from build123d import *

# Parameters (mm, degrees)
F0_W          = 30
F0_H          = 30
F4_DEPTH      = 3
F3_W          = 30
F3_H          = 30
F5_DEPTH      = 8
F6_DEPTH      = 25
F8_DEPTH      = 6.0000000522
F10_DEPTH     = 30
F7_W          = 10
F7_H          = 11.7721162952
F7_H_2        = 1.030384494
F11_DEPTH     = 35.21044533
F12_T4_DEPTH  = 18.4976166065
F12_T10_DEPTH = 18.4976166065
F12_T15_DEPTH = 17.5385665297
F12_T20_DEPTH = 17.5385665297
F12_T26_DEPTH = 17.5385665297
F12_T31_DEPTH = 17.5385665297
F12_T37_DEPTH = 18.4976166065
F12_T43_DEPTH = 18.4976166065
F12_T45_DEPTH = 13.9174578279
F12_T47_DEPTH = 24
F12_T49_DEPTH = 44.997612514
F12_T54_DEPTH = 3
F12_T60_DEPTH = 3
F3_W_2        = 10
F3_H_2        = 13
F13_DEPTH     = 5.1313021672
F14_DEPTH     = 10.5


# Not quite as in the source:
# - a fillet or chamfer that OpenCascade refuses, or shapes differently, is made with other operations: its cross-section is extruded or revolved along the edge and cut away or added


with BuildPart() as f4:
    # F0 (on Top) → F4 (new body)
    with BuildSketch(Plane.XY):
        with Locations((0, 15)):
            Rectangle(F0_W, F0_H)
    extrude(amount=F4_DEPTH)

    # F3 (on 3pt) → F5 (join)
    with BuildSketch(Plane(origin=(0, 0, 0), x_dir=(-1, 0, 0), z_dir=(0, 0.984807753, 0.1736481777))):
        with Locations((0, 15)):
            Rectangle(F3_W, F3_H)
        Polygon((-14, 2), (-14, 15), (-14, 25), (14, 25), (14, 2), (-4, 2), align=None, mode=Mode.SUBTRACT)
        Polygon((-14, 25), (-14, 15), (-4, 15), (-4, 2), (14, 2), (14, 25), align=None)
    extrude(amount=F5_DEPTH)

    # F0 (on Top) → F6 (cut)
    with BuildSketch(Plane.XY):
        with Locations((0, 15)):
            Rectangle(F0_W, F0_H)
    extrude(amount=-F6_DEPTH, mode=Mode.SUBTRACT)

    # F3 (on 3pt) → F8 (cut)
    with BuildSketch(Plane(origin=(0, 0, 0), x_dir=(-1, 0, 0), z_dir=(0, 0.984807753, 0.1736481777))):
        Polygon((-14, 25), (-14, 15), (-4, 15), (-4, 2), (14, 2), (14, 25), align=None)
    extrude(amount=F8_DEPTH, mode=Mode.SUBTRACT)

    # F9 (on face) → F10 (join, through all)
    with BuildSketch(Plane.YZ.offset(15)):
        Polygon((30, 3), (2.6690166941, 30.9334180117), (7.594431953, 3), align=None)
        with BuildLine():
            ThreePointArc((11.3703802933, 5.5), (10.0848050739, 5.9679111138), (9.4007647872, 7.1527036447))
            Line((9.4007647872, 7.1527036447), (7.6573020205, 17.0403723366))
            ThreePointArc((7.6573020205, 17.0403723366), (8.7131028501, 19.1666972856), (11.0564624317, 18.7863828744))
            Line((11.0564624317, 18.7863828744), (20.7308856563, 8.8987141825))
            ThreePointArc((20.7308856563, 8.8987141825), (21.1449009434, 6.7245737833), (19.3013407511, 5.5))
            Line((19.3013407511, 5.5), (11.3703802933, 5.5))
        make_face(mode=Mode.SUBTRACT)
    extrude(amount=-F10_DEPTH)

    # F7 (on face) → F11 (cut, through all)
    with BuildSketch(Plane(origin=(0, 30, 0), x_dir=(-1, 0, 0), z_dir=(0, 1, 0))):
        with Locations((-9, 8.8860581476)):
            Rectangle(F7_W, F7_H)
        with Locations((-9, 2.484807753)):
            Rectangle(F7_W, F7_H_2)
    extrude(amount=-F11_DEPTH, mode=Mode.SUBTRACT)

    # F12: fillet of radius 3 on 9 edges, made by hand


with BuildPart() as f12_tool2:
    # F12_s3 → F12_t4 (new body)
    with BuildSketch(Plane.XZ.offset(-25.9817706947)):
        with BuildLine():
            ThreePointArc((7, 14.7721162952), (4.8786796564, 13.8934366387), (4, 11.7721162952))
            Line((4, 11.7721162952), (4, 14.7721162952))
            Line((4, 14.7721162952), (7, 14.7721162952))
        make_face()
    extrude(amount=F12_T4_DEPTH)

    split(bisect_by=Plane(origin=(0, 16.8266333185, 16.4637365227), x_dir=(1, 0, 0), z_dir=(0, -0.7147724526, -0.6993570912)), keep=Keep.TOP)

    split(bisect_by=Plane(origin=(0, 15.0397021871, 14.7153437946), x_dir=(1, 0, 0), z_dir=(0, 0.7147724526, 0.6993570912)), keep=Keep.TOP)


with BuildPart() as f4_1:
    add(f4.part)

    # F12_t1: union F12_tool2
    add(f12_tool2.part)


with BuildPart() as f12_tool8:
    # F12_s9 → F12_t10 (new body)
    with BuildSketch(Plane.XZ.offset(-25.9817706947)):
        with BuildLine():
            ThreePointArc((7, 14.7721162952), (4.8786796564, 13.8934366387), (4, 11.7721162952))
            Line((4, 11.7721162952), (4, 14.7721162952))
            Line((4, 14.7721162952), (7, 14.7721162952))
        make_face()
    extrude(amount=F12_T10_DEPTH)

    split(bisect_by=Plane(origin=(0, 10.3404814066, 1.8233058655), x_dir=(1, 0, 0), z_dir=(0, -0.984807753, -0.1736481777)), keep=Keep.TOP)


with BuildPart() as f4_2:
    add(f4_1.part)

    # F12_t7: union F12_tool8
    add(f12_tool8.part)


with BuildPart() as f12_tool13:
    # F12_s14 → F12_t15 (new body)
    with BuildSketch(Plane.XZ.offset(-15.5572567598)):
        with BuildLine():
            ThreePointArc((7, 14.7721162952), (4.8786796564, 13.8934366387), (4, 11.7721162952))
            Line((4, 11.7721162952), (4, 14.7721162952))
            Line((4, 14.7721162952), (7, 14.7721162952))
        make_face()
    extrude(amount=F12_T15_DEPTH)

    split(bisect_by=Plane(origin=(0, 15.0397021871, 14.7153437946), x_dir=(1, 0, 0), z_dir=(0, 0.7147724526, 0.6993570912)), keep=Keep.TOP)


with BuildPart() as f4_3:
    add(f4_2.part)

    # F12_t12: union F12_tool13
    add(f12_tool13.part)


with BuildPart() as f12_tool18:
    # F12_s19 → F12_t20 (new body)
    with BuildSketch(Plane.XZ.offset(-15.5572567598)):
        with BuildLine():
            ThreePointArc((7, 14.7721162952), (4.8786796564, 13.8934366387), (4, 11.7721162952))
            Line((4, 11.7721162952), (4, 14.7721162952))
            Line((4, 14.7721162952), (7, 14.7721162952))
        make_face()
    extrude(amount=F12_T20_DEPTH)

    split(bisect_by=Plane(origin=(0, 10.3404814066, 1.8233058655), x_dir=(1, 0, 0), z_dir=(0, -0.984807753, -0.1736481777)), keep=Keep.TOP)

    split(bisect_by=Plane(origin=(0, 7.8784620241, 1.3891854213), x_dir=(1, 0, 0), z_dir=(0, 0.984807753, 0.1736481777)), keep=Keep.TOP)


with BuildPart() as f4_4:
    add(f4_3.part)

    # F12_t17: union F12_tool18
    add(f12_tool18.part)


with BuildPart() as f12_tool24:
    # F12_s25 → F12_t26 (new body)
    with BuildSketch(Plane.XZ.offset(-15.5572567598)):
        with BuildLine():
            ThreePointArc((14, 11.7721162952), (13.1213203436, 13.8934366387), (11, 14.7721162952))
            Line((11, 14.7721162952), (14, 14.7721162952))
            Line((14, 14.7721162952), (14, 11.7721162952))
        make_face()
    extrude(amount=F12_T26_DEPTH)

    split(bisect_by=Plane(origin=(0, 15.0397021871, 14.7153437946), x_dir=(1, 0, 0), z_dir=(0, 0.7147724526, 0.6993570912)), keep=Keep.TOP)


with BuildPart() as f4_5:
    add(f4_4.part)

    # F12_t23: union F12_tool24
    add(f12_tool24.part)


with BuildPart() as f12_tool29:
    # F12_s30 → F12_t31 (new body)
    with BuildSketch(Plane.XZ.offset(-15.5572567598)):
        with BuildLine():
            ThreePointArc((14, 11.7721162952), (13.1213203436, 13.8934366387), (11, 14.7721162952))
            Line((11, 14.7721162952), (14, 14.7721162952))
            Line((14, 14.7721162952), (14, 11.7721162952))
        make_face()
    extrude(amount=F12_T31_DEPTH)

    split(bisect_by=Plane(origin=(0, 10.3404814066, 1.8233058655), x_dir=(1, 0, 0), z_dir=(0, -0.984807753, -0.1736481777)), keep=Keep.TOP)

    split(bisect_by=Plane(origin=(0, 7.8784620241, 1.3891854213), x_dir=(1, 0, 0), z_dir=(0, 0.984807753, 0.1736481777)), keep=Keep.TOP)


with BuildPart() as f4_6:
    add(f4_5.part)

    # F12_t28: union F12_tool29
    add(f12_tool29.part)


with BuildPart() as f12_tool35:
    # F12_s36 → F12_t37 (new body)
    with BuildSketch(Plane.XZ.offset(-25.9817706947)):
        with BuildLine():
            ThreePointArc((14, 11.7721162952), (13.1213203436, 13.8934366387), (11, 14.7721162952))
            Line((11, 14.7721162952), (14, 14.7721162952))
            Line((14, 14.7721162952), (14, 11.7721162952))
        make_face()
    extrude(amount=F12_T37_DEPTH)

    split(bisect_by=Plane(origin=(0, 16.8266333185, 16.4637365227), x_dir=(1, 0, 0), z_dir=(0, -0.7147724526, -0.6993570912)), keep=Keep.TOP)

    split(bisect_by=Plane(origin=(0, 15.0397021871, 14.7153437946), x_dir=(1, 0, 0), z_dir=(0, 0.7147724526, 0.6993570912)), keep=Keep.TOP)


with BuildPart() as f4_7:
    add(f4_6.part)

    # F12_t34: union F12_tool35
    add(f12_tool35.part)


with BuildPart() as f12_tool41:
    # F12_s42 → F12_t43 (new body)
    with BuildSketch(Plane.XZ.offset(-25.9817706947)):
        with BuildLine():
            ThreePointArc((14, 11.7721162952), (13.1213203436, 13.8934366387), (11, 14.7721162952))
            Line((11, 14.7721162952), (14, 14.7721162952))
            Line((14, 14.7721162952), (14, 11.7721162952))
        make_face()
    extrude(amount=F12_T43_DEPTH)

    split(bisect_by=Plane(origin=(0, 10.3404814066, 1.8233058655), x_dir=(1, 0, 0), z_dir=(0, -0.984807753, -0.1736481777)), keep=Keep.TOP)


with BuildPart() as f4_8:
    add(f4_7.part)

    # F12_t40: union F12_tool41
    add(f12_tool41.part)

    # F12_s46 → F12_t45 (cut)
    with BuildSketch(Plane(origin=(0, -7.3860581476, -1.3023613325), x_dir=(1, 0, 0), z_dir=(0, 0.984807753, 0.1736481777))):
        with BuildLine():
            ThreePointArc((-15, -27), (-14.1213203436, -29.1213203436), (-12, -30))
            Line((-12, -30), (-15, -30))
            Line((-15, -30), (-15, -27))
        make_face()
        with BuildLine():
            ThreePointArc((15, -27), (14.1213203436, -29.1213203436), (12, -30))
            Line((12, -30), (15, -30))
            Line((15, -30), (15, -27))
        make_face()
    extrude(amount=F12_T45_DEPTH, mode=Mode.SUBTRACT)

    # F12_s48 → F12_t47 (cut)
    with BuildSketch(Plane.YZ.offset(-12)):
        with BuildLine():
            ThreePointArc((1.1105168936, 30.6586124474), (2.5491593686, 30.5603807939), (3.7757787843, 29.8022604621))
            Line((3.7757787843, 29.8022604621), (2.6690166941, 30.9334180117))
            Line((2.6690166941, 30.9334180117), (1.1105168936, 30.6586124474))
        make_face()
    extrude(amount=F12_T47_DEPTH, mode=Mode.SUBTRACT)

    # F12_s50 → F12_t49 (cut)
    with BuildSketch(Plane(origin=(0, 18.4185448657, -18.8245299169), x_dir=(1, 0, 0), z_dir=(0, -0.6993570912, 0.7147724526))):
        with BuildLine():
            ThreePointArc((-15, 20.5412448507), (-14.1213203436, 22.6625651943), (-12, 23.5412448507))
            Line((-12, 23.5412448507), (-15, 23.5412448507))
            Line((-15, 23.5412448507), (-15, 20.5412448507))
        make_face()
        with BuildLine():
            ThreePointArc((15, 20.5412448507), (14.1213203436, 22.6625651943), (12, 23.5412448507))
            Line((12, 23.5412448507), (15, 23.5412448507))
            Line((15, 23.5412448507), (15, 20.5412448507))
        make_face()
    extrude(amount=F12_T49_DEPTH, mode=Mode.SUBTRACT)


with BuildPart() as f12_tool52:
    # F12_s53 → F12_t54 (new body)
    with BuildSketch(Plane.YZ.offset(-12)):
        Polygon((1.6314614266, 27.7041891884), (1.1105168936, 30.6586124474), (2.6690166941, 30.9334180117), (3.7757787843, 29.8022604621), align=None)
    extrude(amount=-F12_T54_DEPTH)

    # F12_s55 → F12_t56 (revolve, cut)
    with BuildSketch(Plane(origin=(-12, 1.6314614266, 27.7041891884), x_dir=(0, -0.305899314, -0.9520638685), z_dir=(0, 0.9520638685, -0.305899314))):
        with BuildLine():
            ThreePointArc((0, -3), (3, 0), (0, 3))
            Line((0, 3), (0, -3))
        make_face()
    revolve(axis=Axis((-12, 1.6314614266, 27.7041891884), (-1, 0, 0)), mode=Mode.SUBTRACT)


with BuildPart() as f4_9:
    add(f4_8.part)

    # F12_t51: cut F12_tool52
    add(f12_tool52.part, mode=Mode.SUBTRACT)


with BuildPart() as f12_tool58:
    # F12_s59 → F12_t60 (new body)
    with BuildSketch(Plane.YZ.offset(12)):
        Polygon((1.6314614266, 27.7041891884), (3.7757787843, 29.8022604621), (2.6690166941, 30.9334180117), (1.1105168936, 30.6586124474), align=None)
    extrude(amount=F12_T60_DEPTH)

    # F12_s61 → F12_t62 (revolve, cut)
    with BuildSketch(Plane(origin=(12, 1.6314614266, 27.7041891884), x_dir=(0, -0.305899314, -0.9520638685), z_dir=(0, -0.9520638685, 0.305899314))):
        with BuildLine():
            ThreePointArc((0, -3), (3, 0), (0, 3))
            Line((0, 3), (0, -3))
        make_face()
    revolve(axis=Axis((12, 1.6314614266, 27.7041891884), (1, 0, 0)), mode=Mode.SUBTRACT)


with BuildPart() as f4_10:
    add(f4_9.part)

    # F12_t57: cut F12_tool58
    add(f12_tool58.part, mode=Mode.SUBTRACT)

    # F3 (on 3pt) → F13 (cut, through all)
    with BuildSketch(Plane(origin=(0, 0, 0), x_dir=(-1, 0, 0), z_dir=(0, 0.984807753, 0.1736481777))):
        with Locations((0, 15)):
            Rectangle(F3_W, F3_H)
        Polygon((-14, 2), (-14, 15), (-14, 25), (14, 25), (14, 2), (-4, 2), align=None, mode=Mode.SUBTRACT)
        Polygon((-14, 25), (-14, 15), (-4, 15), (-4, 2), (14, 2), (14, 25), align=None)
        with Locations((-9, 8.5)):
            Rectangle(F3_W_2, F3_H_2)
    extrude(amount=-F13_DEPTH, mode=Mode.SUBTRACT)

    # F3 (on 3pt) → F14 (cut, through all)
    with BuildSketch(Plane(origin=(0, 0, 0), x_dir=(-1, 0, 0), z_dir=(0, 0.984807753, 0.1736481777))):
        with Locations((-9, 8.5)):
            Rectangle(F3_W_2, F3_H_2)
    extrude(amount=F14_DEPTH, mode=Mode.SUBTRACT)


solid = f4_10.part
Can you work these out from the model? Positions are in its coordinate system, mm. A direction names the side the tool comes from. Give positions to 0.01 mm unless a question says otherwise; leave off trailing zeros. Loops run counter-clockwise (first coordinate to the right, second up) from the corner with the lowest first, then second, coordinate; pieces in that order, holes last. Notation, with made-up numbers: M 16,-5 L 45,-5 A13 ccw 45,17 Z; hole C 49.25,-36.5 d10. An arc over 180 degrees is marked long. One line per item, written item: value.
1) Thinking about a two-plate mould opening in X: for faces 4 (the face through (-0.168, 2.53, 30.567)), 5 (the face through (9.1, 5.5, 16.2)), 6 (the face through (-15, 8, 11)), which applies, +X half, -X half, draft (parallel to the pull), parting line (faces both ways), or undercut?
Geometry check:
face 4: draft
face 5: undercut
face 6: -X half
2) Imagine slicing it at A-A on x = 9.5. Write out the boundary of the cut face in (y, z).
Geometry check:
outline: M -5.21,29.54 L -4.34,24.62 L 1.57,25.66 L 3.3,15.81 L 7.74,16.6 L 7.66,17.04 A2 cw 11.06,18.79 L 14.98,14.77 L 18.48,14.77 L 3.78,29.8 A3 ccw 1.11,30.66 Z; M -0.35,1.97 L 0,0 L 30,0 L 30,1.97 Z
3) Please list where these lines run through material, in increasing order: line 1 (X direction, y = -0.5, z = 16.5); line 2 (Z direction, x = -5.5, y = 19.5); line 3 (Z direction, x = -5, y = 15).
Geometry check:
line 1: x = -15 to -14, 14 to 15
line 2: z = 0 to 5.51, 10.16 to 13.73
line 3: z = 0 to 5.5, 14.76 to 18.33
4) I'm going to push flat-ended pins straight in: pin 1 (1.5 mm diameter, centred on x = -5.5, y = 23, fed in from +Z); pin 2 (1.5 mm diameter, centred on x = 2, y = 19, fed in from +Z); pin 3 (8 mm diameter, centred on x = 6.5, y = 10, fed in from +Z); pin 4 (12 mm diameter, centred on x = -4.5, y = 2.5, fed in from -Z). Where does each tip first touch, or does it pass through?
Geometry check:
pin 1: stops at z = 10.92
pin 2: stops at z = 15.01
pin 3: stops at z = 27.53
pin 4: stops at z = 0
5) On a 3-axis mill with a long thin cutter (end or side, diameter ignored), from which of +Z, -Z, +X, -X, +Y, -Y can I reach the whole of each face in a straight line? I mean faces 1 (the face through (14.507, 10.1, 5.955)), 2 (the face through (9, 15, 1.97)), 3 (the face through (-0.196, -1.428, 25.134)). Say none if no direction works.
Geometry check:
face 1: +X, -X
face 2: +Y, -Y
face 3: none
6) Imagine slicing it at B-B on x = -6. Write out the boundary of the cut face in (y, z).
Geometry check:
outline: M -5.21,29.54 L -4.34,24.62 L 1.57,25.66 L 5.56,3.01 L -0.35,1.97 L 0,0 L 30,0 L 30,3 L 3.78,29.8 A3 ccw 1.11,30.66 Z; hole M 7.66,17.04 L 9.4,7.15 A2 ccw 11.37,5.5 L 19.3,5.5 A2 ccw 20.73,8.9 L 11.06,18.79 A2 ccw Z
